For this review, take the finished solid that the model builds, in its own axes (mm). A direction names the side the tool comes from. Coordinates: 2 decimals unless noted, no trailing zeros. Loops run counter-clockwise (first coordinate to the right, second up) from the corner with the lowest first, then second, coordinate; pieces in that order, holes last. Notation, with made-up numbers: M 78,-34 L 136,-34 A14 cw 136,-18 Z; hole C 82,-26.75 d3. An arc over 180 degrees is marked long. Write each question's results on one line, items separated by ' | '. Start each with the question number.
```python
from build123d import *

# Parameters (mm, degrees)
F0_W      = 70
F0_H      = 20
F1_DEPTH  = 6.5
F4_DEPTH  = 4
F5_R      = 2.6
F6_DEPTH  = 13.001
F7_DEPTH  = 13.001
F9_R      = 5
F8_R      = 3.1
F10_DEPTH = 20.001
F11_W     = 45
F11_H     = 11
F12_DEPTH = 0.8
F13_W     = 11
F13_H     = 1.6
F14_DEPTH = 4.5
F15_W     = 14
F15_H     = 1.4
F16_DEPTH = 20.0010001
F17_R     = 4.25
F18_DEPTH = 3.5


with BuildPart() as f1:
    # F0 (on Top) → F1 (new body, symmetric)
    with BuildSketch(Plane.XY):
        Rectangle(F0_W, F0_H)
    extrude(amount=F1_DEPTH, both=True)

    # F3 (on face) → F4 (cut)
    with BuildSketch(Plane.XY.offset(6.5)):
        Polygon((-31, -4.6188021535), (-27, -2.3094010768), (-27, 2.3094010768), (-31, 4.6188021535), (-35, 2.3094010768), (-35, -2.3094010768), align=None)
        Polygon((35, -2.3094010768), (35, 2.3094010768), (31, 4.6188021535), (27, 2.3094010768), (27, -2.3094010768), (31, -4.6188021535), align=None)
    extrude(amount=-F4_DEPTH, mode=Mode.SUBTRACT)

    # F5 (on face) → F6 (cut, through all)
    with BuildSketch(Plane.XY.offset(6.5)):
        with Locations((-31, 0)):
            Circle(F5_R)
        with Locations((31, 0)):
            Circle(F5_R)
    extrude(amount=-F6_DEPTH, mode=Mode.SUBTRACT)

    # F2 (on face) → F7 (cut, through all)
    with BuildSketch(Plane.XY.offset(6.5)):
        with BuildLine():
            Line((-17, -3), (17, -3))
            ThreePointArc((17, -3), (20, 0), (17, 3))
            Line((17, 3), (-17, 3))
            ThreePointArc((-17, 3), (-20, 0), (-17, -3))
        make_face()
    extrude(amount=-F7_DEPTH, mode=Mode.SUBTRACT)

    # F9
    f9_edges = [f1.edges().sort_by_distance(p)[0] for p in [
        (35, -10, 0),
        (-35, -10, 0),
        (35, 10, 0),
        (-35, 10, 0),
    ]]
    fillet(f9_edges, radius=F9_R)

    # F8 (on face) → F10 (cut, through all)
    with BuildSketch(Plane.XZ.offset(10)):
        with Locations((-25.5, -0.5)):
            Circle(F8_R)
        with Locations((25.5, -0.5)):
            Circle(F8_R)
    extrude(amount=-F10_DEPTH, mode=Mode.SUBTRACT)

    # F11 (on Top) → F12 (cut, symmetric)
    with BuildSketch(Plane.XY):
        Rectangle(F11_W, F11_H)
    extrude(amount=F12_DEPTH, both=True, mode=Mode.SUBTRACT)

    # F13 (on face) → F14 (cut, through all)
    with BuildSketch(Plane.XZ.offset(10)):
        Rectangle(F13_W, F13_H)
    extrude(amount=-F14_DEPTH, mode=Mode.SUBTRACT)

    # F15 (on face) → F16 (cut, through all)
    with BuildSketch(Plane.XZ.offset(10)):
        with Locations((-28, -0.2)):
            Rectangle(F15_W, F15_H)
        with Locations((28, -0.2)):
            Rectangle(F15_W, F15_H)
    extrude(amount=-F16_DEPTH, mode=Mode.SUBTRACT)

    # F17 (on face) → F18 (cut)
    with BuildSketch(Plane(origin=(0, 0, -6.5), x_dir=(1, 0, 0), z_dir=(0, 0, -1))):
        with Locations((31, 0)):
            Circle(F17_R)
        with Locations((-31, 0)):
            Circle(F17_R)
    extrude(amount=-F18_DEPTH, mode=Mode.SUBTRACT)


solid = f1.part
```
Q1. Take a section at B-B, the plane y = -7.25. Give the boundary of the cut face in (x, z).
Q2. Take a section at C-C, the plane z = -4.5. Give the boundary of the cut face in (x, y), then the cut area to 3 significant figures.
Q3. Take a section at A-A, the plane z = 3.5. Give the boundary of the cut face in (x, y).
Q4. Insertion check: P1, Ø7, axis at x = -31, y = 0, coming from the -Z side; P2, Ø3, axis at x = 31, y = 0, coming from the -Z side (3 decimals); P3, Ø1.8, axis at y = -8.5, z = 0, coming from the +X side. Each pin has a flat end and moves straight along its axis. Give the tip position at first contact, or say it passes through.
Q5. For faces 1 (the face through (27, 0, 5)), 2 (the face through (-32.97, 3.48, 4.53)), 3 (the face through (21, -7, 0)), 4 (the face through (-26.753, 0.166, -4.774)), 5 (the face through (0, -4, 0.8)), list the 3-axis set-ups (+Z, -Z, +X, -X, +Y, -Y) from which the entire face can be reached by the end or side of a thin tool; tool diameter is ignored.
Q6. To check wall thickness, follow line 1 along Y through (x, z) = (-11, -5); line 2 along X through (y, z) = (0, -1.5); line 3 along X through (y, z) = (0, -4.75). State the ranges of each line that lie inside material, in increasing order.
Q7. The part is to be moulded in two halves that separate along Z. For faces 6 (the face through (33, -2, -3)), 7 (the face through (25.4, -0.1, -3.6)), 8 (the face through (-25.4, -0.1, 2.6)), 9 (the face through (-20, 0, -4)), say which applies: pulls with the +Z half, pulls with the -Z half, needs draft (parallel to the pull), parting line crosses it, or undercut.
Q8. Take a section at D-D, the plane y = 8.25. Give the boundary of the cut face in (x, z).
Results:
1) outline: M -34.47,-6.5 L 34.47,-6.5 L 34.47,-0.9 L 28.57,-0.9 A3.1 cw 22.43,-0.9 L 21,-0.9 L 21,0.5 L 22.57,0.5 A3.1 cw 28.43,0.5 L 34.47,0.5 L 34.47,6.5 L -34.47,6.5 L -34.47,0.5 L -28.43,0.5 A3.1 cw -22.57,0.5 L -21,0.5 L -21,-0.9 L -22.43,-0.9 A3.1 cw -28.57,-0.9 L -34.47,-0.9 Z; hole M -5.5,-0.8 L 5.5,-0.8 L 5.5,0.8 L -5.5,0.8 Z
2) outline: M -35,-5 A5 ccw -30,-10 L 30,-10 A5 ccw 35,-5 L 35,-1.44 A4.25 cw long 35,1.44 L 35,5 A5 ccw 30,10 L -30,10 A5 ccw -35,5 L -35,1.44 A4.25 cw long -35,-1.44 Z; hole M -17,-3 L 17,-3 A3 ccw 17,3 L -17,3 A3 ccw Z | area: 1,030 mm^2
3) outline: M -35,-5 A5 ccw -30,-10 L 30,-10 A5 ccw 35,-5 L 35,-2.31 L 31,-4.62 L 27,-2.31 L 27,2.31 L 31,4.62 L 35,2.31 L 35,5 A5 ccw 30,10 L -30,10 A5 ccw -35,5 L -35,2.31 L -31,4.62 L -27,2.31 L -27,-2.31 L -31,-4.62 L -35,-2.31 Z; hole M -17,-3 L 17,-3 A3 ccw 17,3 L -17,3 A3 ccw Z
4) P1: z = -3 | P2: through | P3: x = 34.17
5) face 1: +Z, +X | face 2: +Z | face 3: +X, +Y, -Y | face 4: -Z | face 5: none
6) line 1: -10 to -3, 3 to 10 | line 2: -35 to -33.6, -22.57 to -20, 20 to 22.57, 33.6 to 35 | line 3: -26.75 to -20, 20 to 26.75
7) face 6: pulls with the -Z half | face 7: undercut | face 8: undercut | face 9: needs draft
8) outline: M -33.8,-6.5 L 33.8,-6.5 L 33.8,-0.9 L 28.57,-0.9 A3.1 cw 22.43,-0.9 L 21,-0.9 L 21,0.5 L 22.57,0.5 A3.1 cw 28.43,0.5 L 33.8,0.5 L 33.8,6.5 L -33.8,6.5 L -33.8,0.5 L -28.43,0.5 A3.1 cw -22.57,0.5 L -21,0.5 L -21,-0.9 L -22.43,-0.9 A3.1 cw -28.57,-0.9 L -33.8,-0.9 Z
